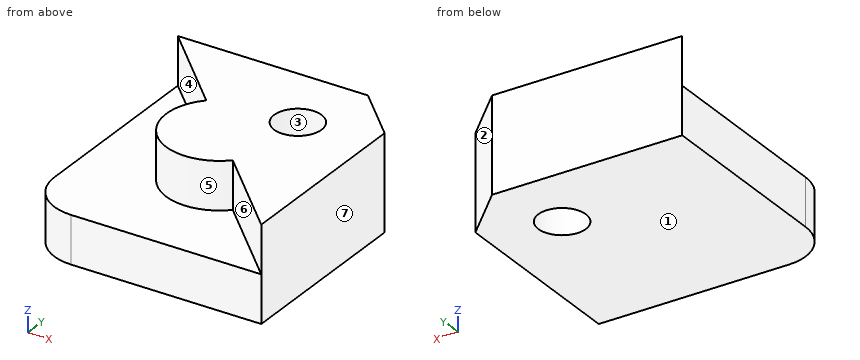
```python
from build123d import *

# Parameters (mm, degrees)
F0_W     = 25
F0_H     = 25
F1_DEPTH = 5
F3_DEPTH = 5
F4_R     = 5
F5_SIZE  = 5
F7_DEPTH = 5
F8_R     = 2.5
F9_DEPTH = 10.001


with BuildPart() as f1:
    # F0 (on Top) → F1 (new body)
    with BuildSketch(Plane.XY):
        Rectangle(F0_W, F0_H)
    extrude(amount=F1_DEPTH)

    # F2 (on face) → F3 (join)
    with BuildSketch(Plane.XY.offset(5)):
        Polygon((12.5, 12.5), (-12.5, 12.5), (12.5, -12.5), align=None)
    extrude(amount=F3_DEPTH)

    # F4
    f4_edges = [f1.edges().sort_by_distance(p)[0] for p in [
        (-12.5, -12.5, 2.5),
    ]]
    fillet(f4_edges, radius=F4_R)

    # F5
    f5_edges = [f1.edges().sort_by_distance(p)[0] for p in [
        (12.5, 12.5, 5),
    ]]
    chamfer(f5_edges, length=F5_SIZE)

    # F6 (on face) → F7 (join)
    with BuildSketch(Plane.XY.offset(5)):
        with BuildLine():
            Line((3.9644660941, -3.9644660941), (-3.9644660941, 3.9644660941))
            ThreePointArc((-3.9644660941, 3.9644660941), (-3.9644660941, -3.9644660941), (3.9644660941, -3.9644660941))
        make_face()
    extrude(amount=F7_DEPTH)

    # F8 (on face) → F9 (cut, through all)
    with BuildSketch(Plane.XY.offset(10)):
        with Locations((5, 5)):
            Circle(F8_R)
    extrude(amount=-F9_DEPTH, mode=Mode.SUBTRACT)


solid = f1.part
```
The listing builds one solid part. Answer for the finished solid, in the listing's coordinates (mm). Face numbers are marked on the shaded views. A direction names the side the tool comes from. Round coordinates to 2 decimals unless told otherwise and drop trailing zeros. Loops run counter-clockwise (first coordinate to the right, second up) from the corner with the lowest first, then second, coordinate; pieces in that order, holes last. Notation, with made-up numbers: (69, 21.5) - (80, 21.5) arc R22 ccw to (80, 40.5) - close; hole circle Ø6 at (3, -33.5). An arc over 180 degrees is marked (long way). Use one line per item in the form item = value. Start each with the question number.
1. The part is cut by section D-D on x = -6.25. Determine the outline of the cut face in (y, z).
2. Given pin 1 Ø2 at (x, z) = (9, 7.5) entering from +Y, flat-ended and moving along its own axis, determine where the tip first touches the part or whether it passes through.
3. Consider line 1 (Y direction, x = 5, z = 2.5); line 2 (Z direction, x = -9, y = -7.75); line 3 (Y direction, x = 5, z = 7). Determine where each line is inside the solid, lowest interval first. Write a range as [from, to].
4. For a pull along X with two mould halves and no side action, classify the marked faces 1, 2 and 3 as pulls with the +X half, pulls with the -X half, needs draft (parallel to the pull), parting line crosses it, or undercut.
5. The part is cut by section A-A on y = 5. Determine the outline of the cut face in (x, z), then the cut area to 4 significant figures.
6. A tool of negligible diameter and unlimited length cuts with its end or side. For the marked faces 4, 5, 6 and 7, from which of +Z, -Z, +X, -X, +Y, -Y can it reach the whole face along a straight path? Write none if from no direction.
Geometry check:
q1.outline = (-12.5, 0) - (12.5, 0) - (12.5, 10) - (6.25, 10) - (6.25, 5) - (-12.5, 5) - close
q2.pin_1 = 12
q3.line_1 = [-12.5, 2.5], [7.5, 12.5]
q3.line_2 = [0, 5]
q3.line_3 = [-5, 2.5], [7.5, 12.5]
q4.face_1 = needs draft
q4.face_2 = pulls with the +X half
q4.face_3 = undercut
q5.outline = (-12.5, 0) - (2.5, 0) - (2.5, 10) - (-5, 10) - (-5, 5) - (-12.5, 5) - close; (7.5, 0) - (12.5, 0) - (12.5, 10) - (7.5, 10) - close
q5.area = 162.5 mm^2
q6.face_4 = +Z, -X
q6.face_5 = +Z
q6.face_6 = +Z, -Y
q6.face_7 = +Z, -Z, +X, +Y, -Y
